Work out the finished part from the listing and answer in its coordinate system (mm). A direction names the side the tool comes from. Coordinates: 2 decimals unless noted, no trailing zeros. Loops run counter-clockwise (first coordinate to the right, second up) from the corner with the lowest first, then second, coordinate; pieces in that order, holes last. Notation, with made-up numbers: (87.25, 45.5) -> (105.25, 45.5) arc R23 ccw to (105.25, 75.5) -> close; hole circle Ø7 at (52, 66.5). An arc over 180 degrees is marked (long way). One line per question, with ' | ' between items.
Autodesk Inventor part; units mm, degrees
ref_plane "Work Plane1" through (164.5, 127, 270) normal (1, 0, 0) x (0, 0, 1)
ref_plane "XZ Plane" through (0, 0, 0) normal (0, 1, 0) x (-1, 0, 0)
ref_plane "XY Plane" through (0, 0, 0) normal (0, 0, 1) x (1, 0, 0)
sketch "Sketch1" plane through (0, 0, 0) normal (0, 0, 1) x (1, 0, 0)
  line L0 (0, 0) -> (100, 0)
  line L1 (100, 0) -> (100, 25)
  line L2 (100, 25) -> (0, 25)
  line L3 (0, 25) -> (0, 0)
  line L4 (0, 25) -> (115.2078, 140.2078)
  line L5 (100, 0) -> (177.7078, 77.7078)
  line L6 (151.2922, 176.2922) -> (200.5844, 163.0844)
  line L7 (200.5844, 163.0844) -> (213.7922, 113.7922)
  line L8 (213.7922, 113.7922) -> (177.7078, 77.7078)
  line L9 (177.7078, 77.7078) -> (128.4156, 90.9156)
  line L10 (128.4156, 90.9156) -> (115.2078, 140.2078)
  line L11 (115.2078, 140.2078) -> (151.2922, 176.2922)
  circle A0 centre (164.5, 127) radius 4
  dimension "d0" = 100
  dimension "d1" = 25
  dimension "d6" = 8
  dimension "d8" = 45
  dimension "d15" = 127
extrude "Extrusion1" add sketch "Sketch1" along normal blind 20
sketch "Sketch2" plane through (0, 0, 20) normal (0, 0, 1) x (1, 0, 0)
  line L0 (0, 25) -> (0, 0)
  line L1 (0, 0) -> (100, 0)
  line L2 (0, 25) -> (100, 25)
  line L3 (100, 25) -> (100, 0)
  line L4 (100, 0) -> (0, 0)
  line L5 (0, 0) -> (0, 25)
  line L6 (100, 25) -> (125, 25)
  line L7 (100, 0) -> (213.7922, 113.7922)
  line L8 (100, 0) -> (125, 25)
extrude "Extrusion2" add sketch "Sketch2" along normal blind 250
sketch "Sketch4" plane through (0, 0, 270) normal (0, 0, 1) x (1, 0, 0)
  line L0 (0, 25) -> (125, 25)
  line L1 (125, 25) -> (213.7922, 113.7922)
  line L2 (213.7922, 113.7922) -> (200.5844, 163.0844)
  line L3 (200.5844, 163.0844) -> (151.2922, 176.2922)
  line L4 (151.2922, 176.2922) -> (0, 25)
  circle A0 centre (164.5, 127) radius 4
  line L5 (100, 0) -> (125, 25)
  line L6 (125, 25) -> (0, 25)
  line L7 (0, 25) -> (0, 0)
  line L8 (0, 0) -> (100, 0)
extrude "Extrusion3" add sketch "Sketch4" along normal blind 20
sketch "Sketch5" plane through (0, 0, 0) normal (0, -1, 0) x (1, 0, 0)
  line L0 (0, 0) -> (100, 0)
  line L1 (100, 0) -> (100, 290)
  line L2 (0, 290) -> (100, 290)
  line L3 (0, 0) -> (0, 290)
  line L4 (0, 0) -> (-125.5737, 72.5)
  line L5 (-125.5737, 72.5) -> (-125.5737, 217.5)
  line L6 (-125.5737, 217.5) -> (0, 290)
  line L7 (0, 290) -> (125.5737, 217.5)
  line L8 (125.5737, 217.5) -> (125.5737, 72.5)
  line L9 (125.5737, 72.5) -> (0, 0)
  point P0 (0, 145)
extrude "Extrusion4" add sketch "Sketch5" against normal blind 25 contours L4 L5 L6 L3
sketch "Sketch6" plane through (0, 25, 20) normal (0, 1, 0) x (1, 0, 0)
  line L0 (100, 20) -> (100, -270)
  circle A0 centre (-24.528, -125) radius 3
  circle A1 centre (-31.528, -125) radius 1.5
  circle A2 centre (-21.028, -131.0622) radius 1.5
  circle A3 centre (-21.028, -118.9378) radius 1.5
  point P0 (0, 20)
  point P1 (100, -125)
  dimension "d18" = 6
  dimension "d19" = 124.528
  dimension "d20" = 3
  dimension "d21" = 7
  dimension "d24" = 360
extrude "Extrusion5" cut sketch "Sketch6" against normal through all
sketch "Sketch7" plane through (100, 0, 0) normal (0, -1, 0) x (1, 0, 0)
  circle A0 centre (-124.528, 145) radius 3
  circle A1 centre (-124.528, 145) radius 12
  point P0 (-100, 0)
  dimension "d28" = 24
extrude "Extrusion6" cut sketch "Sketch7" against normal blind 5
sketch "Sketch8" plane through (0, 0, 270) normal (0, 0, -1) x (-1, 0, 0)
  circle A0 centre (-164.5, 127) radius 4
  circle A1 centre (-164.5, 127) radius 12.5
  point P0 (0, 0)
  dimension "d31" = 25
extrude "Extrusion7" cut sketch "Sketch8" against normal blind 7
sketch "Sketch10" plane through (164.5, 127, 277) normal (0, 0, -1) x (-1, 0, 0)
  circle A0 centre (7, 0) radius 2
  circle A1 centre (0, 0) radius 4
  circle A2 centre (-3.5, 6.0622) radius 2
  circle A3 centre (-3.5, -6.0622) radius 2
  point P0 (164.5, -127)
  dimension "d34" = 4
  dimension "d37" = 360
  dimension "d39" = 7
extrude "Extrusion8" cut sketch "Sketch10" against normal through all
sketch "Sketch11" plane through (0, 0, 290) normal (0, 0, 1) x (1, 0, 0)
  circle A0 centre (168, 133.0622) radius 2
  circle A1 centre (164.5, 127) radius 4
  circle A2 centre (168, 133.0622) radius 4
  circle A3 centre (157.5, 127) radius 4
  circle A4 centre (168, 120.9378) radius 4
  point P0 (0, 0)
  dimension "d42" = 8
  dimension "d45" = 360
extrude "Extrusion9" cut sketch "Sketch11" against normal blind 3 contours A0 | A1 A4 A3 A2 | A2 A1 | A1 A2 | A4 A1 | A1 A4 | A3 A1 | A1 A3
ref_plane "Work Plane1" through (164.5, 127, 270) normal (1, 0, 0) x (0, 0, 1)
sketch "Sketch12" plane through (164.5, 127, 270) normal (1, 0, 0) x (0, 0, 1)
  line L0 (17, -1.9365) -> (17, 1.9365)
  line L1 (17, 1.9365) -> (20, 1.9365)
  line L2 (20, 3.9993) -> (20, 1.9365)
  line L3 (20, 3.9993) -> (17, 3.9993)
  line L4 (17, 3.9993) -> (17, 2.0628)
  line L5 (17, 2.0628) -> (20, 2.0628)
  line L6 (20, -2.0628) -> (20, 2.0628)
  line L7 (20, -2.0628) -> (17, -2.0628)
  line L8 (17, -2.0628) -> (17, -3.9993)
  line L9 (17, -3.9993) -> (20, -3.9993)
  line L10 (20, -1.9365) -> (20, -3.9993)
  line L11 (20, -1.9365) -> (17, -1.9365)
  line L12 (7, 4) -> (7, -4)
  line L13 (7, -12.5) -> (7, 12.5)
  line L14 (0, -12.5) -> (0, 12.5)
  circle A0 centre (3.5, 0) radius 2
  line L15 (0, -12.5) -> (7, -12.5)
  point P0 (-270, 127)
  point P1 (7, 0)
  point P2 (3.5, -12.5)
  dimension "d50" = 4
extrude "Extrusion10" cut sketch "Sketch12" along normal through all contours A0
sketch "Sketch13" plane through (0, 0, 290) normal (0, 0, 1) x (1, 0, 0)
  line L0 (100, 0) -> (213.7922, 113.7922)
  line L1 (213.7922, 113.7922) -> (200.5844, 163.0844)
  line L2 (200.5844, 163.0844) -> (151.2922, 176.2922)
  line L3 (151.2922, 176.2922) -> (0, 25)
  line L4 (0, 25) -> (0, 0)
  line L5 (0, 0) -> (100, 0)
  arc A0 (161, 128.9365) -> (161, 125.0635) centre (157.5, 127) ccw
  arc A1 (164.5729, 130.9993) -> (161, 128.9365) centre (164.5, 127) ccw
  arc A2 (167.9271, 129.0628) -> (164.5729, 130.9993) centre (168, 133.0622) ccw
  arc A3 (167.9271, 124.9372) -> (167.9271, 129.0628) centre (164.5, 127) ccw
  arc A4 (164.5729, 123.0007) -> (167.9271, 124.9372) centre (168, 120.9378) ccw
  arc A5 (161, 125.0635) -> (164.5729, 123.0007) centre (164.5, 127) ccw
extrude "Extrusion11" cut sketch "Sketch13" against normal blind 20 contours L5 L4 L3 L2 L1 L0 | A1 A2 A3 A4 A5 A0
sketch "Sketch14" plane through (0, 0, 0) normal (0, 0, -1) x (-1, 0, 0)
  circle A0 centre (-164.5, 127) radius 4
  line L0 (0, 0) -> (-100, 0)
  line L1 (0, 25) -> (0, 0)
  line L2 (-151.2922, 176.2922) -> (0, 25)
  line L3 (-200.5844, 163.0844) -> (-151.2922, 176.2922)
  line L4 (-213.7922, 113.7922) -> (-200.5844, 163.0844)
  line L5 (-100, 0) -> (-213.7922, 113.7922)
extrude "Extrusion12" cut sketch "Sketch14" against normal blind 20
sketch "Sketch15" plane through (0, 0, 20) normal (0, 0, -1) x (-1, 0, 0)
  circle A0 centre (-90, 12.5) radius 2.5
  circle A1 centre (-15, 12.5) radius 2.5
  line L0 (-90, 12.5) -> (-15, 12.5) construction
  line L1 (0, 0) -> (-100, 0)
  dimension "d57" = 5
  dimension "d58" = 5
  dimension "d59" = 75
  dimension "d60" = 12.5
  dimension "d61" = 10
extrude "Extrusion13" cut sketch "Sketch15" against normal through all
sketch "Sketch16" plane through (-125.5737, 25, 217.5) normal (0, 1, 0) x (1, 0, 0)
  circle A0 centre (101.0457, 72.5) radius 22.5
  circle A1 centre (101.0457, 72.5) radius 3 construction
  point P0 (125.5737, 217.5)
  dimension "d64" = 45
extrude "Extrusion14" cut sketch "Sketch16" against normal through all
sketch "Sketch17" plane through (-125.5737, 25, 217.5) normal (0, 1, 0) x (1, 0, 0)
  circle A0 centre (50.0457, 72.5) radius 2.5
  circle A1 centre (101.0457, 72.5) radius 22.5 construction
  circle A2 centre (75.5457, 28.3327) radius 2.5
  circle A3 centre (126.5457, 28.3327) radius 2.5
  circle A4 centre (152.0457, 72.5) radius 2.5
  circle A5 centre (126.5457, 116.6673) radius 2.5
  circle A6 centre (75.5457, 116.6673) radius 2.5
  point P0 (125.5737, 217.5)
  dimension "d68" = 5
  dimension "d69" = 51
  dimension "d72" = 360
extrude "Extrusion15" cut sketch "Sketch17" against normal through all
properties part number "HA02" material "ABS Plastic"
1) Find section A-A (y = 20.5). Write down the section's boundary in (x, z), plus the area to 3 significant figures.
Check values:
outline: (-125.57, 72.5) -> (0, 0) -> (0, 20) -> (120.5, 20) -> (120.5, 270) -> (0, 270) -> (0, 290) -> (-125.57, 217.5) -> close; hole circle Ø5 at (-75.53, 145); hole circle Ø5 at (-50.03, 100.83); hole circle Ø5 at (-50.03, 189.17); hole circle Ø45 at (-24.53, 145); hole circle Ø5 at (0.97, 100.83); hole circle Ø5 at (0.97, 189.17); hole circle Ø5 at (26.47, 145) | area: 55,700 mm^2
2) Find the intervals of material crossed by line 1 along X through (y, z) = (10.25, 228); line 2 along Z through (x, y) = (-52, 17.75); line 3 along X through (y, z) = (7.75, 143), in increasing order.
Check values:
line 1: x = -107.39 to 13.91, 16.09 to 88.91, 91.09 to 110.25 | line 2: z = 30.02 to 99.3, 102.37 to 187.63, 190.7 to 259.98 | line 3: x = -125.57 to -77.03, -74.03 to -46.94, -2.12 to 24.97, 27.97 to 107.75
3) For faces 4 (the face through (-61.908, 12.325, 35.743)), 5 (the face through (62, 13, 270)), 6 (the face through (0, 13, 10)), determine the directions among +Z, -Z, +X, -X, +Y, -Y from which every point of the face is accessible in a straight line to the end or side of a thin tool.
Check values:
face 4: -Z, -X, +Y, -Y | face 5: +Z, +X, +Y, -Y | face 6: -Z, +X, +Y, -Y
4) Flat-ended cylindrical pins translate along their axes: pin 1 (12 mm diameter, centred on x = -79, y = 21.5, fed in from +Z); pin 2 (10 mm diameter, centred on y = 10, z = 279, fed in from +X); pin 3 (12 mm diameter, centred on x = 97.5, y = 11.5, fed in from +Z). Find the tip coordinate at first contact, or state that the pin passes through.
Check values:
pin 1: stops at z = 247.85 | pin 2: stops at x = 0 | pin 3: stops at z = 270
5) Find section B-B (x = -60). Write down the section's boundary in (y, z).
Check values:
outline: (0, 34.64) -> (25, 34.64) -> (25, 255.36) -> (0, 255.36) -> close
6) The mould has two halves that part along X. Classify faces 1 (the face through (0, 13, 280)), 2 (the face through (-27.46, 12.68, 122.69)), 3 (the face through (49, 13, 20)): released by +X, released by -X, zero draft, split by the parting line, or undercut.
Check values:
face 1: released by +X | face 2: undercut | face 3: zero draft
